```python
from build123d import *

# Parameters (mm, degrees)
LEG_OUTLINE_R = 2.65
LEG_OUTLINE_W = 47.454147397
LEG_OUTLINE_H = 16.449498304
LEG_DEPTH     = 6


# Read off the part's stored shape, not the designer's step: leg
with BuildPart() as part:
    # leg outline → leg (new body)
    with BuildSketch(Plane(origin=(0, 0, 0), x_dir=(1, 0, 0), z_dir=(0, 1, 0))):
        Polygon((0, 0), (330, 0), (330, 134.5), (169.6, 134.5), (169.6, 128.5), (103.5, 128.5), (103.5, 455.5), (73.5, 455.5), (0, 134.5), align=None)
        with Locations((51.75, 6)):
            Circle(LEG_OUTLINE_R, mode=Mode.SUBTRACT)
        with Locations((106.5, 33.625)):
            Circle(LEG_OUTLINE_R, mode=Mode.SUBTRACT)
        with Locations((164.625, 6)):
            Circle(LEG_OUTLINE_R, mode=Mode.SUBTRACT)
        with Locations((106.5, 100.875)):
            Circle(LEG_OUTLINE_R, mode=Mode.SUBTRACT)
        with Locations((171.976991955, 94.176840096)):
            Rectangle(LEG_OUTLINE_W, LEG_OUTLINE_H, mode=Mode.SUBTRACT)
        with Locations((274.875, 6)):
            Circle(LEG_OUTLINE_R, mode=Mode.SUBTRACT)
    extrude(amount=LEG_DEPTH)


solid = part.part
```
Source: CAD feature listing. Evaluate the final solid. Frame: model axes, mm. Give positions to 0.01 mm unless a question says otherwise; leave off trailing zeros. Write each loop counter-clockwise with the first axis right and the second up, starting at its lowest first coordinate (ties: lowest second). Pieces come first, ordered by that corner, then holes.
1. Section query D-D (x = 284.5). Return the cut outline in (y, z).
2. First-contact query: pin 1 (3 mm diameter, centred on y = 4, z = -272, fed in from -X); pin 2 (3 mm diameter, centred on y = 4, z = -229, fed in from +X); pin 3 (1.8 mm diameter, centred on x = 128.5, y = 4, fed in from -Z). Flat tips, straight axial feed; report the tip coordinate or a pass-through.
3. Material intervals for line 1 along X through (y, z) = (4.65, -6) (3 decimals); line 2 along Z through (x, y) = (106.5, 1.6) (3 decimals); line 3 along Z through (x, y) = (161.5, 4), sorted ascending.
4. Section query A-A (x = 177). Return the cut outline in (y, z).
5. Section query C-C (z = -403). Return the cut outline in (x, y), then the cut area to 3 significant figures.
6. Section query B-B (y = 4). Return the cut outline in (x, z) (3 decimals), then the cut area to 3 significant figures.
Output values:
1. outline: (0, -134.5) - (6, -134.5) - (6, 0) - (0, 0) - close
2. pin 1: stops at x = 31.14
2. pin 2: stops at x = 103.5
2. pin 3: stops at z = -128.5
3. line 1: x = 0 to 49.1, 54.4 to 161.975, 167.275 to 272.225, 277.525 to 330
3. line 2: z = -128.5 to -103.525, -98.225 to -36.275, -30.975 to 0
3. line 3: z = -128.5 to -102.4, -85.95 to 0
4. outline: (0, -134.5) - (6, -134.5) - (6, -102.4) - (0, -102.4) - close; (0, -85.95) - (6, -85.95) - (6, 0) - (0, 0) - close
5. outline: (61.48, 0) - (103.5, 0) - (103.5, 6) - (61.48, 6) - close
5. area: 252 mm2
6. outline: (0, -134.5) - (73.5, -455.5) - (103.5, -455.5) - (103.5, -128.5) - (169.6, -128.5) - (169.6, -134.5) - (330, -134.5) - (330, 0) - (0, 0) - close; hole circle Ø5.3 at (51.75, -6); hole circle Ø5.3 at (106.5, -100.875); hole circle Ø5.3 at (106.5, -33.625); hole (148.25, -102.402) - (195.704, -102.402) - (195.704, -85.952) - (148.25, -85.952) - close; hole circle Ø5.3 at (164.625, -6); hole circle Ø5.3 at (274.875, -6)
6. area: 64,500 mm2
